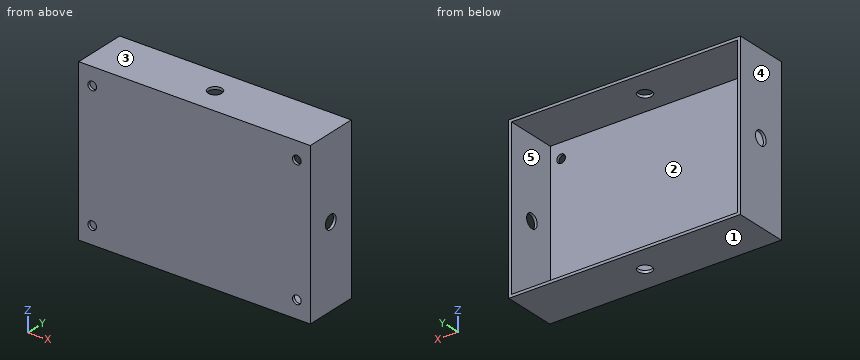
```python
from build123d import *

# Parameters (mm, degrees)
SKETCH_1_W          = 86
SKETCH_1_H          = 60
EXTRUDE_1_DEPTH     = 20
SKETCH_2_W          = 84
SKETCH_2_H          = 58
CUT_EXTRUDE_1_DEPTH = 19
SKETCH_3_R          = 1.6
CUT_EXTRUDE_2_DEPTH = 1
SKETCH_4_R          = 2.6
CUT_EXTRUDE_3_DEPTH = 94.252345815
SKETCH_5_R          = 2.6
CUT_EXTRUDE_4_DEPTH = 77.47875522


with BuildPart() as part:
    # 草图1 → 凸台-拉伸1 (new body)
    with BuildSketch(Plane(origin=(0, 0, 0), x_dir=(1, 0, 0), z_dir=(0, 1, 0))):
        Rectangle(SKETCH_1_W, SKETCH_1_H)
    extrude(amount=EXTRUDE_1_DEPTH)

    # 草图2 → 切除-拉伸1 (cut)
    with BuildSketch(Plane(origin=(0, 20, 0), x_dir=(1, 0, 0), z_dir=(0, 1, 0))):
        Rectangle(SKETCH_2_W, SKETCH_2_H)
    extrude(amount=-CUT_EXTRUDE_1_DEPTH, mode=Mode.SUBTRACT)

    # 草图3 → 切除-拉伸2 (cut)
    with BuildSketch(Plane.XZ):
        with Locations(Location((-38, 23.5, 0), (0, 0, 270))):
            Circle(SKETCH_3_R)
        with Locations(Location((38, 23.5, 0), (0, 0, 90))):
            Circle(SKETCH_3_R)
        with Locations(Location((38, -23.5, 0), (0, 0, 270))):
            Circle(SKETCH_3_R)
        with Locations(Location((-38, -23.5, 0), (0, 0, 90))):
            Circle(SKETCH_3_R)
    extrude(amount=-CUT_EXTRUDE_2_DEPTH, mode=Mode.SUBTRACT)

    # 草图4 → 切除-拉伸3 (cut, through all)
    with BuildSketch(Plane.ZY.offset(43)):
        with Locations((0, 10)):
            Circle(SKETCH_4_R)
    extrude(amount=-CUT_EXTRUDE_3_DEPTH, mode=Mode.SUBTRACT)

    # 草图5 → 切除-拉伸4 (cut, through all)
    with BuildSketch(Plane(origin=(0, 0, -30), x_dir=(-1, 0, 0), z_dir=(0, 0, -1))):
        with Locations((0, 10)):
            Circle(SKETCH_5_R)
    extrude(amount=-CUT_EXTRUDE_4_DEPTH, mode=Mode.SUBTRACT)


solid = part.part
```
For this review, take the finished solid that the model builds, in its own axes (mm). Face numbers are marked on the shaded views. A direction names the side the tool comes from. Coordinates: 2 decimals unless noted, no trailing zeros. Loops run counter-clockwise (first coordinate to the right, second up) from the corner with the lowest first, then second, coordinate; pieces in that order, holes last.
1. For the marked faces 1 and 2, list the 3-axis set-ups (+Z, -Z, +X, -X, +Y, -Y) from which the entire face can be reached by the end or side of a thin tool; tool diameter is ignored.
2. Add section D-D, the plane z = 8. Give the boundary of the cut face in (x, y).
3. Add section A-A, the plane x = 0. Give the boundary of the cut face in (y, z), then the cut area to 3 significant figures.
4. Insertion check: P1, Ø2.5, axis at x = -38, z = -23.5, coming from the +Y side; P2, Ø10, axis at x = 20, z = 5, coming from the +Y side. Each pin has a flat end and moves straight along its axis. Give the tip position at first contact, or say it passes through.
5. Add section C-C, the plane y = 18.5. Give the boundary of the cut face in (x, z).
6. Add section B-B, the plane z = 23.5. Give the boundary of the cut face in (x, y).
7. For line 1 (X direction, y = 12.75, z = -22); line 2 (Z direction, x = 15, y = 16.25); line 3 (Y direction, x = -42.5, z = 0), list the stretches that pass through material, from the lowest coordinate up.
8. Mouldability with a two-part tool opening along X and no side actions: class the marked faces 3, 4 and 5 as +X half, -X half, draft (parallel to the pull), parting line (faces both ways), or undercut.
Result:
1. face 1: -Z, +X, -X, +Y, -Y
1. face 2: +Y
2. outline: (-43, 0) - (43, 0) - (43, 20) - (42, 20) - (42, 1) - (-42, 1) - (-42, 20) - (-43, 20) - close
3. outline: (0, -30) - (7.4, -30) - (7.4, -29) - (1, -29) - (1, 29) - (7.4, 29) - (7.4, 30) - (0, 30) - close; (12.6, -30) - (20, -30) - (20, -29) - (12.6, -29) - close; (12.6, 29) - (20, 29) - (20, 30) - (12.6, 30) - close
3. area: 87.6 mm2
4. P1: passes through
4. P2: stops at y = 1
5. outline: (-43, -30) - (43, -30) - (43, 30) - (-43, 30) - close; hole (-42, -29) - (42, -29) - (42, 29) - (-42, 29) - close
6. outline: (-43, 0) - (-39.6, 0) - (-39.6, 1) - (-42, 1) - (-42, 20) - (-43, 20) - close; (-36.4, 0) - (36.4, 0) - (36.4, 1) - (-36.4, 1) - close; (39.6, 0) - (43, 0) - (43, 20) - (42, 20) - (42, 1) - (39.6, 1) - close
7. line 1: x = -43 to -42, 42 to 43
7. line 2: z = -30 to -29, 29 to 30
7. line 3: y = 0 to 7.4, 12.6 to 20
8. face 3: draft
8. face 4: -X half
8. face 5: undercut
